Model file for the job. Use its own axes, mm. Face numbers are marked on the shaded views. A direction names the side the tool comes from. Coordinates: 2 decimals unless noted, no trailing zeros. Write each loop counter-clockwise with the first axis right and the second up, starting at its lowest first coordinate (ties: lowest second). Pieces come first, ordered by that corner, then holes.
Q1. Band-saw the part on A-A, the plane y = -41.5. Write the cut outline in (x, z).
Q2. Band-saw the part on C-C, the plane x = 38. Write the cut outline in (y, z).
Q3. Pull direction Y, two halves, no side cores. Call the marked faces 1, 2, 3 and 4: released by +Y, released by -Y, zero draft, split by the parting line, or undercut.
Q4. Which spindle directions (+Z, -Z, +X, -X, +Y, -Y) get a long thin tool onto all of the face, cutting with end or side? Do the marked faces 5 and 6. Say none if no direction does.
Q5. Band-saw the part on D-D, the plane y = -20. Write the cut outline in (x, z).
Q6. Band-saw the part on B-B, the plane z = -15. Write the cut outline in (x, y).
Q7. Pin check, flat tips, straight feed: P1, Ø1, axis at x = 27, z = 36.5, coming from the -Y side; P2, Ø16.5, axis at x = 0, z = -40, coming from the -Y side; P3, Ø0.9, axis at x = -7, y = -54, coming from the -Z side. Stop position of each tip, or through.
Q8. Drill centre lines: probe 1 along Y at (x, z) = (-47, 60); probe 2 along X at (y, z) = (-6.5, -12.5); probe 3 along Z at (x, y) = (0, -1). Where is each one in solid material? Low to high.
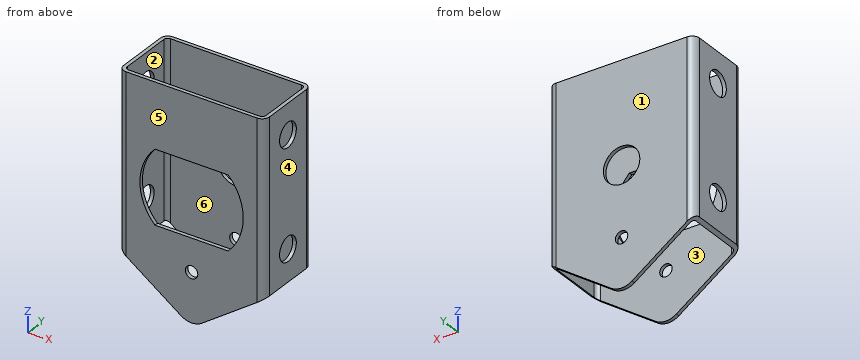
from build123d import *

# Parameters (mm, degrees)
F0_R     = 5.1
F1_DEPTH = 56
F3_DEPTH = 180.001
F5_DEPTH = 3
F6_R     = 15
F7_DEPTH = 25
F8_R     = 10
F9_DEPTH = 120.001
F10_R    = 6


with BuildPart() as f1:
    # F0 (on Front) → F1 (new body)
    with BuildSketch(Plane.XZ):
        with BuildLine():
            Line((60, 100), (-60, 100))
            Line((-60, 100), (-60, -41.2991665388))
            Line((-60, -41.2991665388), (-8.6036465453, -77.2872806643))
            ThreePointArc((-8.6036465453, -77.2872806643), (0, -80), (8.6036465453, -77.2872806643))
            Line((8.6036465453, -77.2872806643), (60, -41.2991665388))
            Line((60, -41.2991665388), (60, 100))
        make_face()
        with Locations((0, -40)):
            Circle(F0_R, mode=Mode.SUBTRACT)
    extrude(amount=F1_DEPTH)

    # F2 (on face) → F3 (cut, through all)
    with BuildSketch(Plane.XY.offset(100)):
        with BuildLine():
            Line((54, -3), (-54, -3))
            ThreePointArc((-54, -3), (-56.1213203436, -3.8786796564), (-57, -6))
            Line((-57, -6), (-57, -50))
            ThreePointArc((-57, -50), (-56.1213203436, -52.1213203436), (-54, -53))
            Line((-54, -53), (54, -53))
            ThreePointArc((54, -53), (56.1213203436, -52.1213203436), (57, -50))
            Line((57, -50), (57, -6))
            ThreePointArc((57, -6), (56.1213203436, -3.8786796564), (54, -3))
        make_face()
    extrude(amount=-F3_DEPTH, mode=Mode.SUBTRACT)

    # F4 (on face) → F5 (cut, through all)
    with BuildSketch(Plane.XZ.offset(56)):
        with BuildLine():
            Line((30.103986447, 47), (-30.103986447, 47))
            ThreePointArc((-30.103986447, 47), (-42.5, 17), (-30.103986447, -13))
            Line((-30.103986447, -13), (30.103986447, -13))
            ThreePointArc((30.103986447, -13), (42.5, 17), (30.103986447, 47))
        make_face()
    extrude(amount=-F5_DEPTH, mode=Mode.SUBTRACT)

    # F6 (on face) → F7 (cut)
    with BuildSketch(Plane.XZ.offset(3)):
        with Locations((0, 17.0000000293)):
            Circle(F6_R)
    extrude(amount=-F7_DEPTH, mode=Mode.SUBTRACT)

    # F8 (on face) → F9 (cut, through all)
    with BuildSketch(Plane.YZ.offset(60)):
        with Locations((-28, 75)):
            Circle(F8_R)
        with Locations((-28, -15)):
            Circle(F8_R)
    extrude(amount=-F9_DEPTH, mode=Mode.SUBTRACT)

    # F10
    f10_edges = [f1.edges().sort_by_distance(p)[0] for p in [
        (-60, -56, 29.350417),
        (60, -56, 29.350417),
        (-60, 0, 29.350417),
        (60, 0, 29.350417),
    ]]
    fillet(f10_edges, radius=F10_R)


solid = f1.part
Answer sheet:
1. outline: (-60, -41.3) - (-57, -43.4) - (-57, 100) - (-60, 100) - close; (57, -43.4) - (60, -41.3) - (60, 100) - (57, 100) - close
2. outline: (-56, -56.7) - (-53, -56.7) - (-53, -2.03) - (-56, -2.03) - close; (-56, 36.03) - (-53, 36.03) - (-53, 100) - (-56, 100) - close; (-3, -56.7) - (0, -56.7) - (0, 100) - (-3, 100) - close
3. face 1: released by +Y
3. face 2: undercut
3. face 3: undercut
3. face 4: zero draft
4. face 5: +Z, -Z, +X, -X, -Y
4. face 6: +Z, -Z
5. outline: (-60, -41.3) - (-57, -43.4) - (-57, -21) - (-60, -21) - close; (-60, -9) - (-57, -9) - (-57, 69) - (-60, 69) - close; (-60, 81) - (-57, 81) - (-57, 100) - (-60, 100) - close; (57, -43.4) - (60, -41.3) - (60, -21) - (57, -21) - close; (57, -9) - (60, -9) - (60, 69) - (57, 69) - close; (57, 81) - (60, 81) - (60, 100) - (57, 100) - close
6. outline: (-60, -50) arc R6 ccw to (-54, -56) - (54, -56) arc R6 ccw to (60, -50) - (60, -38) - (57, -38) - (57, -50) arc R3 cw to (54, -53) - (-54, -53) arc R3 cw to (-57, -50) - (-57, -38) - (-60, -38) - close; (-60, -18) - (-57, -18) - (-57, -6) arc R3 cw to (-54, -3) - (54, -3) arc R3 cw to (57, -6) - (57, -18) - (60, -18) - (60, -6) arc R6 ccw to (54, 0) - (-54, 0) arc R6 ccw to (-60, -6) - close
7. P1: stops at y = -3
7. P2: stops at y = -56
7. P3: stops at z = -78.49
8. probe 1: y = -56 to -53, -3 to 0
8. probe 2: x = -60 to -57, 57 to 60
8. probe 3: z = -80 to -45.1, -34.9 to 2, 32 to 100
